For this review, take the finished solid that the model builds, in its own axes (mm). Give positions to 0.01 mm unless a question says otherwise; leave off trailing zeros. Order: outer loops, then holes, each group sorted by start corner. A loop starts at its lowest first (then second) coordinate and runs counter-clockwise, first axis right, second up. Notation, with made-up numbers: (63.25, -5) - (86.25, -5) arc R32 cw to (86.25, 21) - close; hole circle Ø9 at (-29.5, 26.25). An arc over 180 degrees is marked (long way). Answer as a JSON object with one key per item and string values. Group by question number.
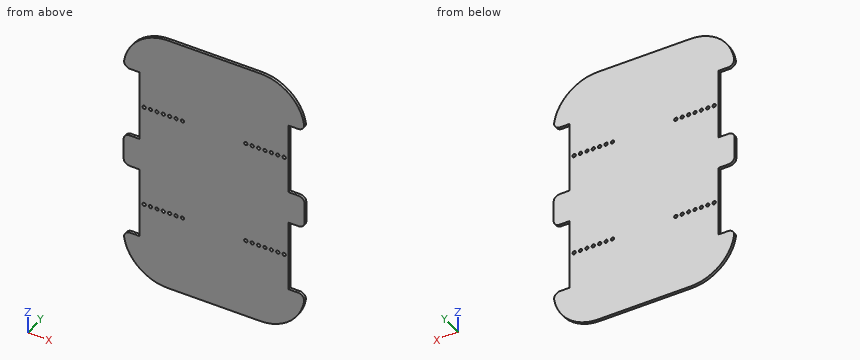
from build123d import *

# Parameters (mm, degrees)
BOSS_EXTRUDE4_DEPTH = 2.8
SKETCH5_R           = 1.65
CUT_EXTRUDE1_DEPTH  = 3.8


with BuildPart() as part:
    # Sketch2 → Boss-Extrude4 (new body)
    with BuildSketch(Plane(origin=(0, 0, 0), x_dir=(1, 0, 0), z_dir=(0, 1, 0))):
        with BuildLine():
            Line((46, -130), (-46, -130))
            ThreePointArc((-46, -130), (-74.550970119, -119.478980051), (-89.448061775, -92.947368421))
            ThreePointArc((-89.448061775, -92.947368421), (-88.08864154, -88.106685893), (-83.523326079, -86))
            Line((-83.523326079, -86), (-74, -86))
            Line((-74, -86), (-74, -16))
            Line((-74, -16), (-84, -16))
            ThreePointArc((-84, -16), (-88.242640687, -14.242640687), (-90, -10))
            Line((-90, -10), (-90, 10))
            ThreePointArc((-90, 10), (-88.242640687, 14.242640687), (-84, 16))
            Line((-84, 16), (-74, 16))
            Line((-74, 16), (-74, 86))
            Line((-74, 86), (-83.523326079, 86))
            ThreePointArc((-83.523326079, 86), (-88.08864154, 88.106685893), (-89.448061775, 92.947368421))
            ThreePointArc((-89.448061775, 92.947368421), (-74.550970119, 119.478980051), (-46, 130))
            Line((-46, 130), (46, 130))
            ThreePointArc((46, 130), (74.550970119, 119.478980051), (89.448061775, 92.947368421))
            ThreePointArc((89.448061775, 92.947368421), (88.08864154, 88.106685893), (83.523326079, 86))
            Line((83.523326079, 86), (74, 86))
            Line((74, 86), (74, 16))
            Line((74, 16), (84, 16))
            ThreePointArc((84, 16), (88.242640687, 14.242640687), (90, 10))
            Line((90, 10), (90, -10))
            ThreePointArc((90, -10), (88.242640687, -14.242640687), (84, -16))
            Line((84, -16), (74, -16))
            Line((74, -16), (74, -86))
            Line((74, -86), (83.523326079, -86))
            ThreePointArc((83.523326079, -86), (88.08864154, -88.106685893), (89.448061775, -92.947368421))
            ThreePointArc((89.448061775, -92.947368421), (74.550970119, -119.478980051), (46, -130))
        make_face()
    extrude(amount=BOSS_EXTRUDE4_DEPTH)

    # Sketch5 → Cut-Extrude1 (cut, through all)
    with BuildSketch(Plane(origin=(0, 2.8, 0), x_dir=(1, 0, 0), z_dir=(0, 1, 0))):
        with Locations((-69.6, -51)):
            Circle(SKETCH5_R)
        with Locations((-63.25, -51)):
            Circle(SKETCH5_R)
        with Locations((-56.9, -51)):
            Circle(SKETCH5_R)
        with Locations((-50.55, -51)):
            Circle(SKETCH5_R)
        with Locations((-44.2, -51)):
            Circle(SKETCH5_R)
        with Locations((-37.85, -51)):
            Circle(SKETCH5_R)
        with Locations((-31.5, -51)):
            Circle(SKETCH5_R)
        with Locations((31.5, -51)):
            Circle(SKETCH5_R)
        with Locations((37.85, -51)):
            Circle(SKETCH5_R)
        with Locations((44.2, -51)):
            Circle(SKETCH5_R)
        with Locations((50.55, -51)):
            Circle(SKETCH5_R)
        with Locations((56.9, -51)):
            Circle(SKETCH5_R)
        with Locations((63.25, -51)):
            Circle(SKETCH5_R)
        with Locations((69.6, -51)):
            Circle(SKETCH5_R)
        with Locations((69.6, 51)):
            Circle(SKETCH5_R)
        with Locations((63.25, 51)):
            Circle(SKETCH5_R)
        with Locations((56.9, 51)):
            Circle(SKETCH5_R)
        with Locations((50.55, 51)):
            Circle(SKETCH5_R)
        with Locations((44.2, 51)):
            Circle(SKETCH5_R)
        with Locations((37.85, 51)):
            Circle(SKETCH5_R)
        with Locations((31.5, 51)):
            Circle(SKETCH5_R)
        with Locations((-31.5, 51)):
            Circle(SKETCH5_R)
        with Locations((-37.85, 51)):
            Circle(SKETCH5_R)
        with Locations((-44.2, 51)):
            Circle(SKETCH5_R)
        with Locations((-50.55, 51)):
            Circle(SKETCH5_R)
        with Locations((-56.9, 51)):
            Circle(SKETCH5_R)
        with Locations((-63.25, 51)):
            Circle(SKETCH5_R)
        with Locations((-69.6, 51)):
            Circle(SKETCH5_R)
    extrude(amount=-CUT_EXTRUDE1_DEPTH, mode=Mode.SUBTRACT)


solid = part.part
1) Consider section B-B (z = 66). Give the boundary of the cut face in (x, y), plus the area to 3 significant figures.
2) Consider section A-A (y = 0.6). Give the number of separate pieces and of enclosed holes in the cut face, plus the area to 3 significant figures.
3) For line 1 (Z direction, x = -44.2, y = 1); line 2 (Z direction, x = 57, y = 1.6); line 3 (X direction, y = 2.7, z = -18), list the stretches that pass through material, from the lowest coordinate up.
4) For pin 1 (1 mm diameter, centred on y = 1, z = 15.5, fed in from +X); pin 2 (2 mm diameter, centred on x = 69.6, z = -51, fed in from +Y); pin 3 (0.8 mm diameter, centred on x = 79.5, y = 1, fed in from +Z), all flat-tipped, find the tip position at first contact; note any pin that passes through.
Result set:
{
 "1": {"outline": "(-74, 0) - (74, 0) - (74, 2.8) - (-74, 2.8) - close", "area": "414 mm2"},
 "2": {"separate pieces": "1", "enclosed holes": "28", "area": "40,300 mm2"},
 "3": {"line 1": "z = -130 to -52.65, -49.35 to 49.35, 52.65 to 130", "line 2": "z = -128.6 to -52.65, -49.35 to 49.35, 52.65 to 128.6", "line 3": "x = -74 to 74"},
 "4": {"pin 1": "stops at x = 87.32", "pin 2": "passes through", "pin 3": "stops at z = 114.99"}
}
